Verification items for this drawing (mm, ordinates from the low corner). Round coordinates to 2 decimals unless told otherwise and drop trailing zeros. Order: outer loops, then holes, each group sorted by start corner. A loop starts at its lowest first (then second) coordinate and runs counter-clockwise, first axis right, second up.
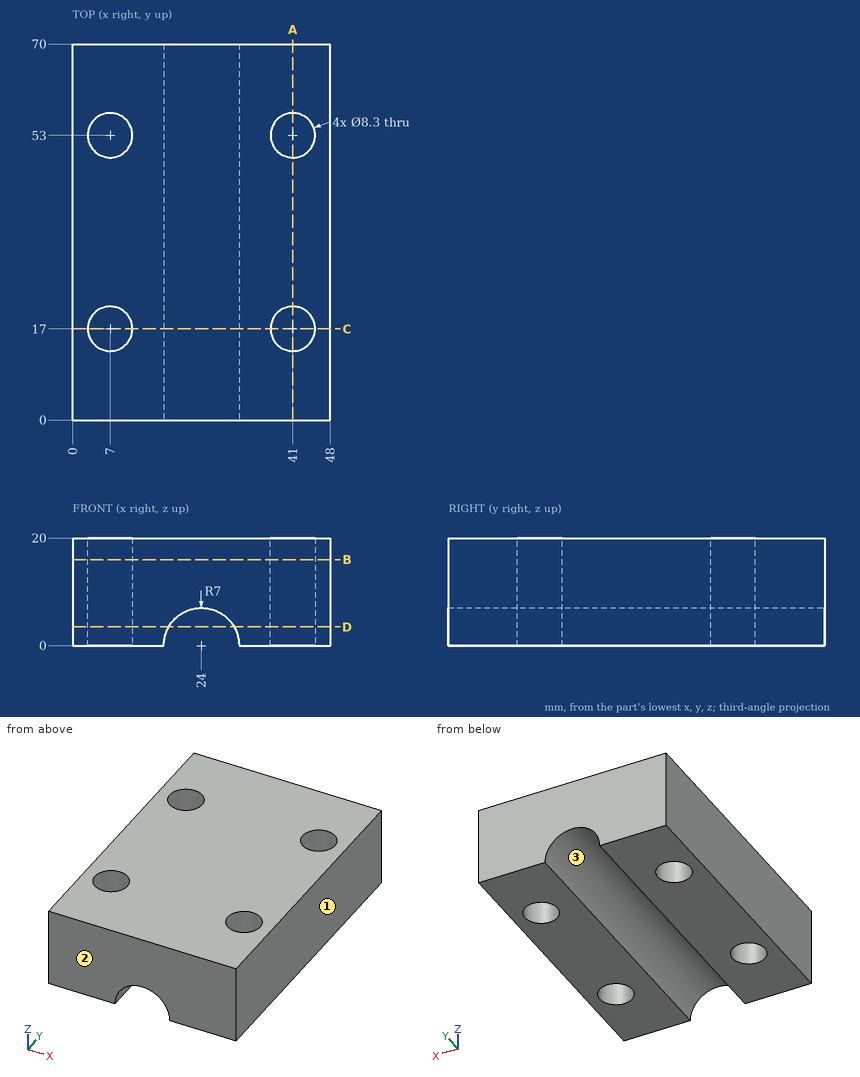
Item 1: Sectioned sample at D-D (z = 3.5). Record the cut outline in (x, y), and give its area (3 significant figures).
Answer:
outline: (0, 0) - (17.94, 0) - (17.94, 70) - (0, 70) - close; (30.06, 0) - (48, 0) - (48, 70) - (30.06, 70) - close; hole circle Ø8.3 at (7, 17); hole circle Ø8.3 at (7, 53); hole circle Ø8.3 at (41, 17); hole circle Ø8.3 at (41, 53)
area: 2,290 mm2
Item 2: Sectioned sample at B-B (z = 16). Record the cut outline in (x, y).
Answer:
outline: (0, 0) - (48, 0) - (48, 70) - (0, 70) - close; hole circle Ø8.3 at (7, 17); hole circle Ø8.3 at (7, 53); hole circle Ø8.3 at (41, 17); hole circle Ø8.3 at (41, 53)
Item 3: Sectioned sample at C-C (y = 17). Record the cut outline in (x, z).
Answer:
outline: (0, 0) - (2.85, 0) - (2.85, 20) - (0, 20) - close; (11.15, 0) - (17, 0) arc R7 cw to (31, 0) - (36.85, 0) - (36.85, 20) - (11.15, 20) - close; (45.15, 0) - (48, 0) - (48, 20) - (45.15, 20) - close
Item 4: Release check for a two-part mould opening along X. For the marked faces 1, 2 and 3 record: released by +X, released by -X, zero draft, split by the parting line, or undercut.
Answer:
face 1: released by +X
face 2: zero draft
face 3: undercut
Item 5: Go/stop test with a flat-tipped pin: P1, Ø5, axis at x = 7, y = 53, coming from the +Z side. Record where the tip stops, or that it passes through.
Answer:
P1: passes through
Item 6: Sectioned sample at A-A (x = 41). Record the cut outline in (y, z).
Answer:
outline: (0, 0) - (12.85, 0) - (12.85, 20) - (0, 20) - close; (21.15, 0) - (48.85, 0) - (48.85, 20) - (21.15, 20) - close; (57.15, 0) - (70, 0) - (70, 20) - (57.15, 20) - close
Item 7: Scan lines: line 1 along Y through (x, z) = (7, 14); line 2 along X through (y, z) = (18, 9); line 3 along X through (y, z) = (51.5, 10.5). Record each from-to range of solid material in increasing order.
Answer:
line 1: y = 0 to 12.85, 21.15 to 48.85, 57.15 to 70
line 2: x = 0 to 2.97, 11.03 to 36.97, 45.03 to 48
line 3: x = 0 to 3.13, 10.87 to 37.13, 44.87 to 48
